Part model, mm, in its own coordinate system. Round coordinates to 2 decimals unless told otherwise and drop trailing zeros. Loops run counter-clockwise (first coordinate to the right, second up) from the corner with the lowest first, then second, coordinate; pieces in that order, holes last.
1) Band-saw the part on C-C, the plane y = -158.5. Write the cut outline in (x, z), then the cut area to 3 significant figures.
2) Probe line 1 (X direction, y = 32.5, z = 0.35); line 2 (Y direction, x = -158.5, z = 2); line 3 (Y direction, x = -172.5, z = 1.65). List the from-to ranges inside material, lowest first.
3) Drop flat-ended pins along their axis: P1, Ø1.2, axis at x = 173, z = 2.5, coming from the +Y side; P2, Ø1.5, axis at x = 126.5, z = 1, coming from the -Y side; P3, Ø1.5, axis at y = -13.5, z = 0.5, coming from the -X side. Give the stop position or say it passes through.
4) Band-saw the part on B-B, the plane x = 109.5. Write the cut outline in (y, z).
5) Band-saw the part on D-D, the plane z = 3.2. State how many separate pieces and enclosed holes the cut face has, then the cut area to 3 significant figures.
6) Band-saw the part on A-A, the plane y = -5.5. Write the cut outline in (x, z), then the cut area to 3 significant figures.
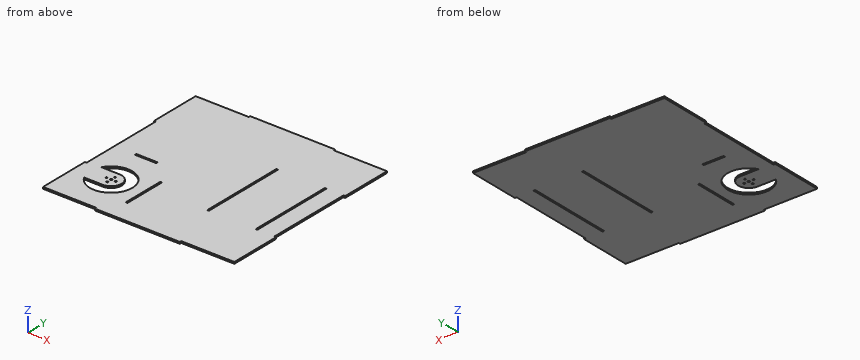
from build123d import *

# Parameters (mm, degrees)
SKETCH1_R           = 2
SKETCH1_R_2         = 2.5
SKETCH1_W           = 50
SKETCH1_H           = 4
SKETCH1_W_2         = 4
SKETCH1_H_2         = 100
SKETCH1_H_3         = 200
BOSS_EXTRUDE1_DEPTH = 4


with BuildPart() as part:
    # Sketch1 → Boss-Extrude1 (new body)
    with BuildSketch(Plane.XY):
        Polygon((-225.544562063, -221.45380172), (-100.544562063, -221.45380172), (-100.544562063, -225.45380172), (99.455437937, -225.45380172), (99.455437937, -221.45380172), (224.455437937, -221.45380172), (224.455437937, -100.45380172), (220.455437937, -100.45380172), (220.455437937, 99.54619828), (224.455437937, 99.54619828), (224.455437937, 220.54619828), (99.455437937, 220.54619828), (99.455437937, 224.54619828), (-100.544562063, 224.54619828), (-100.544562063, 220.54619828), (-225.544562063, 220.54619828), (-225.544562063, 99.54619828), (-221.544562063, 99.54619828), (-221.544562063, -100.45380172), (-225.544562063, -100.45380172), align=None)
        with Locations((-135.544562063, -121.45380172)):
            Circle(SKETCH1_R, mode=Mode.SUBTRACT)
        with Locations((-146.544562063, -110.45380172)):
            Circle(SKETCH1_R, mode=Mode.SUBTRACT)
        with Locations((-157.544562063, -121.45380172)):
            Circle(SKETCH1_R, mode=Mode.SUBTRACT)
        with Locations((-146.544562063, -132.45380172)):
            Circle(SKETCH1_R, mode=Mode.SUBTRACT)
        with Locations((-146.544562063, -121.45380172)):
            Circle(SKETCH1_R_2, mode=Mode.SUBTRACT)
        with BuildLine():
            Line((-146.544562063, -96.45380172), (-189.845832253, -96.45380172))
            ThreePointArc((-189.845832253, -96.45380172), (-96.544562063, -121.45380172), (-189.845832253, -146.45380172))
            Line((-189.845832253, -146.45380172), (-146.544562063, -146.45380172))
            ThreePointArc((-146.544562063, -146.45380172), (-121.544562063, -121.45380172), (-146.544562063, -96.45380172))
        make_face(mode=Mode.SUBTRACT)
        with Locations((-146.544562063, -19.45380172)):
            Rectangle(SKETCH1_W, SKETCH1_H, mode=Mode.SUBTRACT)
        with Locations((-69.544562063, -121.45380172)):
            Rectangle(SKETCH1_W_2, SKETCH1_H_2, mode=Mode.SUBTRACT)
        with Locations((64.455437937, -0.45380172)):
            Rectangle(SKETCH1_W_2, SKETCH1_H_3, mode=Mode.SUBTRACT)
        with Locations((178.455437937, -0.45380172)):
            Rectangle(SKETCH1_W_2, SKETCH1_H_3, mode=Mode.SUBTRACT)
    extrude(amount=BOSS_EXTRUDE1_DEPTH)


solid = part.part
Reported:
1. outline: (-225.54, 0) - (-180.12, 0) - (-180.12, 4) - (-225.54, 4) - close; (-112.97, 0) - (-71.54, 0) - (-71.54, 4) - (-112.97, 4) - close; (-67.54, 0) - (224.46, 0) - (224.46, 4) - (-67.54, 4) - close
1. area: 1,520 mm2
2. line 1: x = -221.54 to 62.46, 66.46 to 176.46, 180.46 to 220.46
2. line 2: y = -221.45 to -170, -146.45 to -123.21, -119.7 to -96.45, -72.9 to -21.45, -17.45 to 220.55
2. line 3: y = -221.45 to -164.19, -146.45 to -96.45, -78.72 to 220.55
3. P1: stops at y = 220.55
3. P2: stops at y = -221.45
3. P3: stops at x = -221.54
4. outline: (-221.45, 0) - (220.55, 0) - (220.55, 4) - (-221.45, 4) - close
5. separate pieces: 1
5. enclosed holes: 10
5. area: 192,000 mm2
6. outline: (-221.54, 0) - (62.46, 0) - (62.46, 4) - (-221.54, 4) - close; (66.46, 0) - (176.46, 0) - (176.46, 4) - (66.46, 4) - close; (180.46, 0) - (220.46, 0) - (220.46, 4) - (180.46, 4) - close
6. area: 1,740 mm2
